```python
from build123d import *

# Parameters (mm, degrees)
F0_W      = 100
F0_H      = 75
F0_W_2    = 90
F0_H_2    = 65
F1_DEPTH  = 50
F2_W      = 2.1659184247
F2_H      = 70.2909231186
F3_DEPTH  = 3
F5_W      = 97.8340815753
F5_H      = 1.5
F6_DEPTH  = 3
F7_W      = 97.8340815753
F7_H      = 1.5
F8_DEPTH  = 3
F9_W      = 100
F9_H      = 75
F9_W_2    = 90
F9_H_2    = 65
F10_DEPTH = 2
F11_W     = 80
F11_H     = 40
F12_DEPTH = 25
F13_R     = 5
F14_DEPTH = 25


with BuildPart() as f1:
    # F0 (on Top) → F1 (new body)
    with BuildSketch(Plane.XY):
        with Locations((6.7471247166, 4.5040409956)):
            Rectangle(F0_W, F0_H)
        with Locations((6.7471247166, 4.5040409956)):
            Rectangle(F0_W_2, F0_H_2, mode=Mode.SUBTRACT)
    extrude(amount=F1_DEPTH)

    # F2 (on face) → F3 (join)
    with BuildSketch(Plane(origin=(0, 0, 0), x_dir=(1, 0, 0), z_dir=(0, 0, -1))):
        Polygon((56.7471247166, 32.9959590044), (-43.2528752834, 32.9959590044), (-43.2528752834, 30.8131203055), (54.5812062919, 30.8131203055), (56.7471247166, 30.8131203055), align=None)
        with Locations((55.6641655043, -4.3323412538)):
            Rectangle(F2_W, F2_H)
        Polygon((54.5812062919, -39.4778028131), (-43.2528752834, -39.4778028131), (-43.2528752834, -42.0040409956), (56.7471247166, -42.0040409956), (56.7471247166, -39.4778028131), align=None)
    extrude(amount=F3_DEPTH)

    # F5 (on face) → F6 (join)
    with BuildSketch(Plane(origin=(0, -30.8131203055, 0), x_dir=(-1, 0, 0), z_dir=(0, 1, 0))):
        with Locations((-5.6641655043, -2.25)):
            Rectangle(F5_W, F5_H)
    extrude(amount=F6_DEPTH)

    # F7 (on face) → F8 (join)
    with BuildSketch(Plane.XZ.offset(-39.4778028131)):
        with Locations((5.6641655043, -2.0621294)):
            Rectangle(F7_W, F7_H)
    extrude(amount=F8_DEPTH)

    # F9 (on face) → F10 (join)
    with BuildSketch(Plane.XY.offset(50)):
        with Locations((6.7471247166, 4.5040409956)):
            Rectangle(F9_W, F9_H)
        with Locations((6.7471247166, 4.5040409956)):
            Rectangle(F9_W_2, F9_H_2, mode=Mode.SUBTRACT)
        with Locations((6.7471247166, 4.5040409956)):
            Rectangle(F9_W_2, F9_H_2)
    extrude(amount=F10_DEPTH)

    # F11 (on face) → F12 (cut)
    with BuildSketch(Plane.XZ.offset(32.9959590044)):
        with Locations((6.7471247166, 25)):
            Rectangle(F11_W, F11_H)
    extrude(amount=-F12_DEPTH, mode=Mode.SUBTRACT)

    # F13 (on face) → F14 (cut)
    with BuildSketch(Plane.YZ.offset(56.7471247166)):
        with Locations((4.5040409956, 32)):
            Circle(F13_R)
    extrude(amount=-F14_DEPTH, mode=Mode.SUBTRACT)


solid = f1.part
```
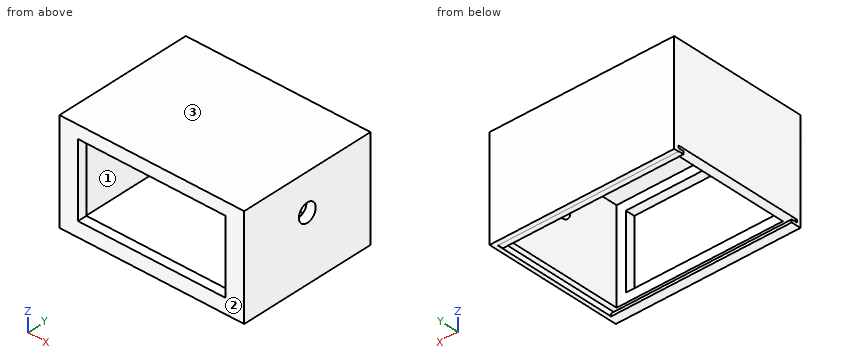
For this review, take the finished solid that the model builds, in its own axes (mm). Face numbers are marked on the shaded views. Coordinates: 2 decimals unless noted, no trailing zeros. Write each loop counter-clockwise with the first axis right and the second up, starting at its lowest first coordinate (ties: lowest second). Pieces come first, ordered by that corner, then holes. Notation, with made-up numbers: (-36.75, -9.5) - (-27.75, -9.5) arc R11 ccw to (-27.75, 1.5) - close; hole circle Ø5 at (1.25, 77). An arc over 180 degrees is marked (long way). Put each result on its own line as item: value.
1. Mouldability with a two-part tool opening along Y and no side actions: class the marked faces 1, 2 and 3 as released by +Y, released by -Y, zero draft, split by the parting line, or undercut.
Values found:
face 1: undercut
face 2: released by -Y
face 3: zero draft
2. Wall thickness on probe 1 along Z at (x, y) = (39, -29); probe 2 along X at (y, z) = (35.5, 1.5); probe 3 along Y at (x, z) = (-20, 2): over which ranges is each line inside the solid? List them lowest first.
Values found:
probe 1: -3 to -1.5, 0 to 5, 45 to 52
probe 2: -43.25 to -38.25, 51.75 to 56.75
probe 3: -33 to -28, 37 to 42
3. Add section C-C, the plane y = 32. Give the boundary of the cut face in (x, z).
Values found:
outline: (-43.25, 0) - (-38.25, 0) - (-38.25, 50) - (51.75, 50) - (51.75, 0) - (54.58, 0) - (54.58, -3) - (56.75, -3) - (56.75, 52) - (-43.25, 52) - close
4. Add section B-B, the plane z = 32. Give the boundary of the cut face in (x, y), then the cut area to 3 significant figures.
Values found:
outline: (-43.25, -33) - (-33.25, -33) - (-33.25, -28) - (-38.25, -28) - (-38.25, 37) - (51.75, 37) - (51.75, 9.5) - (56.75, 9.5) - (56.75, 42) - (-43.25, 42) - close; (46.75, -33) - (56.75, -33) - (56.75, -0.5) - (51.75, -0.5) - (51.75, -28) - (46.75, -28) - close
area: 1,200 mm²
5. For pin 1 (3.5 mm diameter, centred on x = 30, y = 37.5, fed in from -Z); pin 2 (8 mm diameter, centred on x = 1, y = -15.5, fed in from -Z), all flat-tipped, find the tip position at first contact; note any pin that passes through.
Values found:
pin 1: z = -2.81
pin 2: z = 50
6. Add section A-A, the plane x = 0.5. Give the boundary of the cut face in (y, z), then the cut area to 3 significant figures.
Values found:
outline: (-33, -3) - (-27.81, -3) - (-27.81, -1.5) - (-30.81, -1.5) - (-30.81, 0) - (-28, 0) - (-28, 5) - (-33, 5) - close; (-33, 45) - (-28, 45) - (-28, 50) - (37, 50) - (37, 0) - (39.48, 0) - (39.48, -1.31) - (36.48, -1.31) - (36.48, -2.81) - (39.48, -2.81) - (39.48, -3) - (42, -3) - (42, 52) - (-33, 52) - close
area: 473 mm²
7. Add section D-D, the plane z = 25. Give the boundary of the cut face in (x, y).
Values found:
outline: (-43.25, -33) - (-33.25, -33) - (-33.25, -28) - (-38.25, -28) - (-38.25, 37) - (51.75, 37) - (51.75, -28) - (46.75, -28) - (46.75, -33) - (56.75, -33) - (56.75, 42) - (-43.25, 42) - close
